Geometry check sheet. Reference: the model listing, model coordinates, mm. Face numbers are marked on the shaded views. A direction names the side the tool comes from. Round coordinates to 2 decimals unless told otherwise and drop trailing zeros. Loops run counter-clockwise (first coordinate to the right, second up) from the corner with the lowest first, then second, coordinate; pieces in that order, holes last. Notation, with made-up numbers: M 14.25,75 L 67.25,75 A23 cw 67.25,109 Z; hole C 3.5,-38 d11. An arc over 180 degrees is marked long. Answer in a Markdown table with one row per item. Add a question column.
```python
from build123d import *

# Parameters (mm, degrees)
SKETCH_8_W                = 70
SKETCH_8_H                = 30
EXTRUDE_3_DEPTH           = 34.57
SKETCH_9_W                = 30
SKETCH_9_H                = 14.57
SKETCH_9_W_2              = 20
CUT_EXTRUDE_3_DEPTH       = 67.664217758
OTHER_1_OUTLINE_R         = 5.5
OTHER_1_DEPTH             = 5
HOLE_WIZARD_2_D           = 4.5
HOLE_WIZARD_2_DEPTH       = 10
HOLE_WIZARD_2_CBORE_D     = 8
HOLE_WIZARD_2_CBORE_DEPTH = 4.6
BACK_REACH                = 69.458
SKETCH_16_W               = 70
SKETCH_16_H               = 8.975361008
MM_1_D                    = 4
MM_1_DEPTH                = 5
MM_1_TIP                  = 1.201721238
CUT_EXTRUDE_5_DEPTH       = 5
SKETCH_24_W               = 5
SKETCH_24_H               = 21.024638992
SKETCH_24_W_2             = 20
CUT_EXTRUDE_6_DEPTH       = 10
HOLE_WIZARD_3_D           = 6.6
HOLE_WIZARD_3_DEPTH       = 10
HOLE_WIZARD_3_CBORE_D     = 11
HOLE_WIZARD_3_CBORE_DEPTH = 6.8
FILLET_1_R                = 2
SKETCH_29_W               = 10
SKETCH_29_H               = 2
EXTRUDE_5_DEPTH           = 2.329281552
FILLET_3_R                = 2
CUT_EXTRUDE_7_DEPTH       = 0.5
EXTRUDE_START             = 5.016506595
EXTRUDE_6_DEPTH           = 5.016506595
SKETCH_33_R               = 4
CUT_EXTRUDE_8_DEPTH       = 24.57
CUT_EXTRUDE_9_DEPTH       = 67.093990688


# Read off the part's stored shape, not the designer's step: 孔1
with BuildPart() as part:
    # 草图8 → 凸台-拉伸3 (new body)
    with BuildSketch(Plane(origin=(0, 0, 0), x_dir=(1, 0, 0), z_dir=(0, 1, 0))):
        with Locations((13.466824006, -16.724598186)):
            Rectangle(SKETCH_8_W, SKETCH_8_H)
    extrude(amount=EXTRUDE_3_DEPTH)

    # 草图9 → 切除-拉伸3 (cut, through all)
    with BuildSketch(Plane.XY.offset(31.724598186)):
        with Locations((-6.533175994, 17.285)):
            Rectangle(SKETCH_9_W, SKETCH_9_H)
        with Locations((38.466824006, 17.285)):
            Rectangle(SKETCH_9_W_2, SKETCH_9_H)
    extrude(amount=-CUT_EXTRUDE_3_DEPTH, mode=Mode.SUBTRACT)

    # 孔1 outline → 孔1 (cut)
    with BuildSketch(Plane(origin=(0, 0, 0), x_dir=(1, 0, 0), z_dir=(0, 1, 0))):
        with Locations((-1.533175994, -21.724598186)):
            Circle(OTHER_1_OUTLINE_R)
    extrude(amount=OTHER_1_DEPTH, mode=Mode.SUBTRACT)

    # 打孔尺寸(%根据)内六角圆柱头螺钉的类型2
    with Locations(Plane(origin=(-1.533175994, 10, 21.724598186), x_dir=(1, 0, 0), z_dir=(0, 1, 0))):
        with Locations((0, 0)):
            CounterBoreHole(HOLE_WIZARD_2_D / 2, HOLE_WIZARD_2_CBORE_D / 2, HOLE_WIZARD_2_CBORE_DEPTH, depth=HOLE_WIZARD_2_DEPTH)

    # back: up to this face of the body (flat: up to its plane)
    back_end = Plane(part.part.faces().sort_by_distance((-6.533175994, 24.57, 16.724598186))[0])
    # 草图16 → back (cut, up to the picked face)
    with BuildSketch(Plane(origin=(0, 0, 0), x_dir=(1, 0, 0), z_dir=(0, 1, 0)), mode=Mode.PRIVATE) as back_sk1:
        with Locations((13.466824006, -6.21227869)):
            Rectangle(SKETCH_16_W, SKETCH_16_H)
    back_tool1 = split(extrude(back_sk1.sketch, amount=BACK_REACH, mode=Mode.PRIVATE), bisect_by=back_end, keep=Keep.BOTH, mode=Mode.PRIVATE)
    add(back_tool1.solids().sort_by(Axis((13.466824, 0, 6.212279), (0, 1, 0)))[0], mode=Mode.SUBTRACT)

    # 大小mm 暗销孔1
    with Locations(Plane(origin=(-1.533175994, 34.57, 11.724598186), x_dir=(0, 0, 1), z_dir=(0, 1, 0))):
        with Locations((0, 0)):
            Hole(MM_1_D / 2, depth=MM_1_DEPTH)
            with Locations((0, 0, -(MM_1_DEPTH + MM_1_TIP / 2))):  # 118° drill point
                Cone(0, MM_1_D / 2, MM_1_TIP, mode=Mode.SUBTRACT)

    # 草图23 → 切除-拉伸5 (cut)
    with BuildSketch(Plane.XZ.offset(-34.57)):
        with BuildLine():
            Line((28.966824006, 9.724598186), (27.966824006, 9.724598186))
            ThreePointArc((27.966824006, 9.724598186), (25.966824006, 11.724598186), (27.966824006, 13.724598186))
            Line((27.966824006, 13.724598186), (28.966824006, 13.724598186))
            ThreePointArc((28.966824006, 13.724598186), (30.966824006, 11.724598186), (28.966824006, 9.724598186))
        make_face()
    extrude(amount=CUT_EXTRUDE_5_DEPTH, mode=Mode.SUBTRACT)

    # 草图24 → 切除-拉伸6 (cut)
    with BuildSketch(Plane(origin=(0, 0, 0), x_dir=(1, 0, 0), z_dir=(0, 1, 0))):
        with Locations((-19.033175994, -21.21227869)):
            Rectangle(SKETCH_24_W, SKETCH_24_H)
        with Locations((38.466824006, -21.21227869)):
            Rectangle(SKETCH_24_W_2, SKETCH_24_H)
    extrude(amount=CUT_EXTRUDE_6_DEPTH, mode=Mode.SUBTRACT)

    # 打孔尺寸(%根据)内六角圆柱头螺钉的类型3
    with Locations(Plane(origin=(-11.533175994, 24.57, 11.724598186), x_dir=(0, 0, -1), z_dir=(0, -1, 0))):
        with Locations((0, 0), (0, 50)):
            CounterBoreHole(HOLE_WIZARD_3_D / 2, HOLE_WIZARD_3_CBORE_D / 2, HOLE_WIZARD_3_CBORE_DEPTH, depth=HOLE_WIZARD_3_DEPTH)

    # 圆角1
    fillet_1_edges = [part.edges().sort_by_distance(p)[0] for p in [
        (-16.533175994, 0, 21.21227869),
        (-16.533175994, 10, 21.21227869),
        (28.466824006, 0, 21.21227869),
        (-21.533175994, 24.57, 16.724598186),
        (48.466824006, 24.57, 16.724598186),
        (8.466824006, 24.57, 21.21227869),
        (28.466824006, 24.57, 21.21227869),
    ]]
    fillet(fillet_1_edges, radius=FILLET_1_R)

    # 草图29 → 凸台-拉伸5 (add)
    with BuildSketch(Plane(origin=(0, 0, 10.699959194), x_dir=(-1, 0, 0), z_dir=(0, 0, -1))):
        with Locations((0, -1)):
            Rectangle(SKETCH_29_W, SKETCH_29_H)
    extrude(amount=-EXTRUDE_5_DEPTH)

    # 圆角3
    fillet_3_edges = [part.edges().sort_by_distance(p)[0] for p in [
        (-5, -2, 11.86459997),
        (5, -2, 11.86459997),
    ]]
    fillet(fillet_3_edges, radius=FILLET_3_R - 0.0001)  # a hair under: the kernel refuses the full size

    # 草图30 → 切除-拉伸7 (cut)
    with BuildSketch(Plane.XY.offset(31.724598186)):
        with BuildLine():
            Line((-14.533175994, 0), (26.466824006, 0))
            ThreePointArc((26.466824006, 0), (27.881037569, 0.585786438), (28.466824006, 2))
            Line((28.466824006, 2), (28.466824006, 22.57))
            ThreePointArc((28.466824006, 22.57), (29.052610444, 23.984213562), (30.466824006, 24.57))
            Line((30.466824006, 24.57), (46.466824006, 24.57))
            ThreePointArc((46.466824006, 24.57), (47.881037569, 25.155786438), (48.466824006, 26.57))
            Line((48.466824006, 26.57), (48.466824006, 34.57))
            Line((48.466824006, 34.57), (-21.533175994, 34.57))
            Line((-21.533175994, 34.57), (-21.533175994, 26.57))
            ThreePointArc((-21.533175994, 26.57), (-20.947389556, 25.155786438), (-19.533175994, 24.57))
            Line((-19.533175994, 24.57), (6.466824006, 24.57))
            ThreePointArc((6.466824006, 24.57), (7.881037569, 23.984213562), (8.466824006, 22.57))
            Line((8.466824006, 22.57), (8.466824006, 10))
            Line((8.466824006, 10), (-14.533175994, 10))
            ThreePointArc((-14.533175994, 10), (-15.947389556, 9.414213562), (-16.533175994, 8))
            Line((-16.533175994, 8), (-16.533175994, 2))
            ThreePointArc((-16.533175994, 2), (-15.947389556, 0.585786438), (-14.533175994, 0))
        make_face()
    extrude(amount=-CUT_EXTRUDE_7_DEPTH, mode=Mode.SUBTRACT)

    # 草图31 → 凸台-拉伸6 (add)
    with BuildSketch(Plane.XY.offset(31.224598186).offset(EXTRUDE_START)):
        with BuildLine():
            Line((-14.533175994, 0), (26.466824006, 0))
            ThreePointArc((26.466824006, 0), (27.881037569, 0.585786438), (28.466824006, 2))
            Line((28.466824006, 2), (28.466824006, 22.57))
            ThreePointArc((28.466824006, 22.57), (29.052610444, 23.984213562), (30.466824006, 24.57))
            Line((30.466824006, 24.57), (46.466824006, 24.57))
            ThreePointArc((46.466824006, 24.57), (47.881037569, 25.155786438), (48.466824006, 26.57))
            Line((48.466824006, 26.57), (48.466824006, 34.57))
            Line((48.466824006, 34.57), (-21.533175994, 34.57))
            Line((-21.533175994, 34.57), (-21.533175994, 26.57))
            ThreePointArc((-21.533175994, 26.57), (-20.947389556, 25.155786438), (-19.533175994, 24.57))
            Line((-19.533175994, 24.57), (6.466824006, 24.57))
            ThreePointArc((6.466824006, 24.57), (7.881037569, 23.984213562), (8.466824006, 22.57))
            Line((8.466824006, 22.57), (8.466824006, 10))
            Line((8.466824006, 10), (-14.533175994, 10))
            ThreePointArc((-14.533175994, 10), (-15.947389556, 9.414213562), (-16.533175994, 8))
            Line((-16.533175994, 8), (-16.533175994, 2))
            ThreePointArc((-16.533175994, 2), (-15.947389556, 0.585786438), (-14.533175994, 0))
        make_face()
    extrude(amount=-EXTRUDE_6_DEPTH)

    # 草图33 → 切除-拉伸8 (cut)
    with BuildSketch(Plane(origin=(0, 34.57, 0), x_dir=(1, 0, 0), z_dir=(0, 1, 0))):
        with Locations(Location((-1.533175994, -21.724598186, 0), (0, 0, 270))):
            Circle(SKETCH_33_R)
    extrude(amount=-CUT_EXTRUDE_8_DEPTH, mode=Mode.SUBTRACT)

    # 草图34 → 切除-拉伸9 (cut, through all)
    with BuildSketch(Plane.XZ.offset(-24.57)):
        with BuildLine():
            Line((-17.033175994, 17.224598186), (-11.533175994, 17.224598186))
            ThreePointArc((-11.533175994, 17.224598186), (-7.644088697, 15.613685483), (-6.033175994, 11.724598186))
            Line((-6.033175994, 11.724598186), (-6.033175994, 6.224598186))
            Line((-6.033175994, 6.224598186), (-17.033175994, 6.224598186))
            Line((-17.033175994, 6.224598186), (-17.033175994, 17.224598186))
        make_face()
    extrude(amount=CUT_EXTRUDE_9_DEPTH, mode=Mode.SUBTRACT)


solid = part.part
```
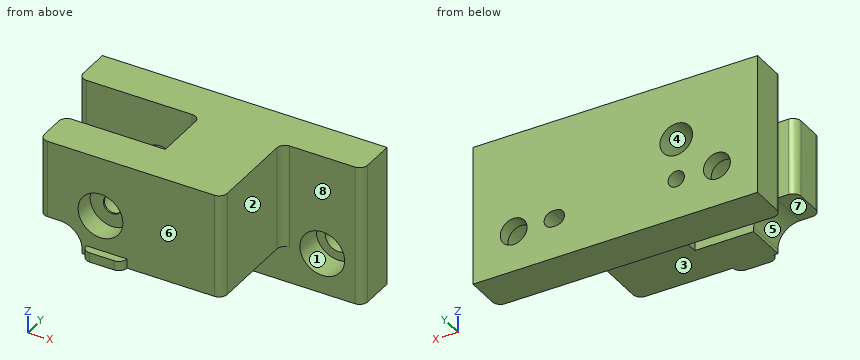
1) Set-up check for the marked faces 1, 2, 3, 4 and 5: record each of +Z, -Z, +X, -X, +Y, -Y from which the full face is reachable in a straight line by a thin tool's end or side.
2) Cross-section at A-A, the plane x = 11. Record the boundary of the cut face in (y, z).
3) Go/stop test with flat-tipped pins: pin 1 (6 mm diameter, centred on y = 14.5, z = 28.5, fed in from +X); pin 2 (9 mm diameter, centred on x = 36, z = 13, fed in from -Y); pin 3 (5 mm diameter, centred on x = -1.53, z = 21.72, fed in from -Y); pin 4 (3 mm diameter, centred on x = 29.5, z = 12.5, fed in from +Y). Record where each tip stops, or that it passes through.
4) Cross-section at B-B, the plane z = 28. Record the boundary of the cut face in (x, y).
5) Thickness scan on L1, parallel to X at y = 26.5, z = 11.5; L2, parallel to X at y = 29.5, z = 9; L3, parallel to Y at x = -7, z = 29. Record the ranges inside material, lowest first. Write a range as [from, to].
6) Draft check along Y on the marked faces 6, 7 and 8. Enter one of: +Y half, -Y half, draft (parallel to the pull), parting line (faces both ways), or undercut.
7) Cross-section at C-C, the plane y = 14. Record the boundary of the cut face in (x, z), plus the area to 3 significant figures.
Worked answers:
| question | item | result |
|---|---|---|
| 1 | face 1 | -Y |
| 1 | face 2 | +Z, -Z, +X, -Y |
| 1 | face 3 | -Z, +X, -X, -Y |
| 1 | face 4 | +Y |
| 1 | face 5 | -Z, -X, -Y |
| 2 | outline | M 0,10.7 L 24.57,10.7 L 24.57,1.72 L 34.57,1.72 L 34.57,36.24 L 0,36.24 Z |
| 3 | pin 1 | stops at x = 28.47 |
| 3 | pin 2 | stops at y = 24.57 |
| 3 | pin 3 | stops at y = 5 |
| 3 | pin 4 | stops at y = 34.57 |
| 4 | outline | M -21.53,26.57 A2 ccw -19.53,24.57 L 6.47,24.57 A2 cw 8.47,22.57 L 8.47,10 L -14.53,10 A2 ccw -16.53,8 L -16.53,2 A2 ccw -14.53,0 L 26.47,0 A2 ccw 28.47,2 L 28.47,22.57 A2 cw 30.47,24.57 L 46.47,24.57 A2 ccw 48.47,26.57 L 48.47,34.57 L -21.53,34.57 Z |
| 5 | L1 | x = [-21.53, -17.03], [-6.04, 32.97], [43.96, 48.47] |
| 5 | L2 | x = [-21.53, -16.31], [-6.76, 33.69], [43.24, 48.47] |
| 5 | L3 | y = [0, 10], [24.57, 34.57] |
| 6 | face 6 | -Y half |
| 6 | face 7 | draft |
| 6 | face 8 | undercut |
| 7 | outline | M 8.47,10.7 L 28.47,10.7 L 28.47,36.24 L 8.47,36.24 Z |
| 7 | area | 511 mm2 |
